Build history of the part. All positions in model axes, mm. Coordinates: 2 decimals unless noted, no trailing zeros. Write each loop counter-clockwise with the first axis right and the second up, starting at its lowest first coordinate (ties: lowest second). Pieces come first, ordered by that corner, then holes. Notation, with made-up numbers: (33, 22.25) -> (50, 22.25) arc R22 cw to (50, 35.25) -> close; hole circle Ø8 at (86, -39.75). An arc over 180 degrees is marked (long way). Write each question's results on one line, items separated by ' | '. Start each with the question number.
Q1. Saw through at C-C on z = 0.95. Give the cut face in (x, y), and give its area (3 significant figures).
Q2. Two-plate mould, pull along X, no slides. Class faces 1 (the face through (10.382, 19.961, 2.096)), 2 (the face through (0, 0, 1.8)), 3 (the face through (-4.63, 20.84, 0.89)), 4 (the face through (0, 0, 3.4)): released by +X, released by -X, zero draft, split by the parting line, or undercut.
Q3. Drop flat-ended pins along their axis: pin 1 Ø21.5 at (x, y) = (-4.5, -4.5) entering from -Z; pin 2 Ø1.5 at (x, z) = (-13.5, 2) entering from -Y; pin 3 Ø1 at (y, z) = (1.5, 2.5) entering from +X. Give the stop position or say it passes through.
Q4. Saw through at A-A on y = 0. Give the cut face in (x, z), and give its area (3 significant figures).
Q5. Drill centre lines: line 1 (Y direction, x = 0, z = 0.5); line 2 (X direction, y = 0.5, z = 1.75); line 3 (Z direction, x = 4, y = 0). Where is each one in solid material? Low to high.
Autodesk Inventor part; units mm, degrees
ref_plane "Arbeitsebene2" through (-21.25, -21.25, 1.8) normal (0, 0, 1) x (1, 0, 0)
ref_plane "YZ Plane" through (0, 0, 0) normal (1, 0, 0) x (0, 1, 0)
ref_plane "XZ Plane" through (0, 0, 0) normal (0, 1, 0) x (-1, 0, 0)
ref_plane "Arbeitsebene1" through (0, 0, 0) normal (0, 0, 1) x (1, 0, 0)
sketch "Skizze1" plane through (0, 0, 0) normal (0, 0, 1) x (1, 0, 0)
  arc A0 (20.5477, -9.1676) -> (20.5477, 9.1676) centre (0, 0) ccw
  arc A1 (20.5477, 9.1676) -> (-20.5477, 9.1676) centre (0, 0) ccw
  arc A2 (-20.5477, 9.1676) -> (-20.5477, -9.1676) centre (0, 0) ccw
  arc A3 (-20.5477, -9.1676) -> (20.5477, -9.1676) centre (0, 0) ccw
  circle A4 centre (0, 0) radius 21.25
  circle A5 centre (0, 0) radius 21.35
  dimension "d0" = 0.1
ref_plane "Arbeitsebene2" through (-21.25, -21.25, 1.8) normal (0, 0, 1) x (1, 0, 0)
extrude "Extrusion1" add sketch "Skizze1" along normal up to surface (1.8 mm away) contours A3 A2 A1 A0
sketch "Skizze2" plane through (0, 0, 1.8) normal (0, 0, 1) x (1, 0, 0)
  circle A0 centre (0, 0) radius 22.5
extrude "Extrusion2" add sketch "Skizze2" along normal blind 1.6
fillet "Rundung1" radius 1 1 edges at (-22.5, 0, 3.4)
properties part number "totmannschalter_deckel"
Returned:
1) outline: circle Ø45 at (0, 0); hole circle Ø42.7 at (0, 0) | area: 158 mm2
2) face 1: split by the parting line | face 2: undercut | face 3: undercut | face 4: zero draft
3) pin 1: stops at z = 1.8 | pin 2: stops at y = -18.54 | pin 3: stops at x = 22.48
4) outline: (-22.5, 0) -> (-21.35, 0) -> (-21.35, 1.8) -> (21.35, 1.8) -> (21.35, 0) -> (22.5, 0) -> (22.5, 2.4) arc R1 ccw to (21.5, 3.4) -> (-21.5, 3.4) arc R1 ccw to (-22.5, 2.4) -> close | area: 75.7 mm2
5) line 1: y = -22.5 to -21.35, 21.35 to 22.5 | line 2: x = -22.49 to -21.34, 21.34 to 22.49 | line 3: z = 1.8 to 3.4
